Work out the finished part from the listing and answer in its coordinate system (mm). A direction names the side the tool comes from. Coordinates: 2 decimals unless noted, no trailing zeros. Write each loop counter-clockwise with the first axis right and the second up, starting at its lowest first coordinate (ties: lowest second). Pieces come first, ordered by that corner, then holes. Notation, with made-up numbers: (-15, 15) - (10, 15) arc R27 cw to (10, 52) - close; hole circle Ø6 at (45.25, 79). An arc over 180 degrees is marked (long way). Answer as a JSON object with one key per item and string values. Group by question number.
from build123d import *

# Parameters (mm, degrees)
F0_W      = 100
F0_H      = 40
F0_R      = 1.5
F1_DEPTH  = 30
F2_W      = 94
F2_H      = 34
F2_R      = 1
F3_DEPTH  = 27
F4_R      = 3
F5_DEPTH  = 5
F6_R      = 1
F7_R      = 4
F8_R      = 4
F9_R      = 6.6732690133
F10_DEPTH = 1
F11_R     = 0.99999


# Not quite as in the source:
# - a fillet or chamfer is up to 0.001 mm smaller than in the source, because OpenCascade refuses the exact size


with BuildPart() as f1:
    # F0 (on Top) → F1 (new body)
    with BuildSketch(Plane.XY):
        with Locations((-4.7806398869, -4.191e-06)):
            Rectangle(F0_W, F0_H)
        with Locations((-21.7806398869, 0)):
            Circle(F0_R, mode=Mode.SUBTRACT)
        with Locations((12.2193601131, 0)):
            Circle(F0_R, mode=Mode.SUBTRACT)
    extrude(amount=F1_DEPTH)

    # F2 (on face) → F3 (cut)
    with BuildSketch(Plane.XY.offset(30)):
        with Locations((-4.7806398869, -4.191e-06)):
            Rectangle(F2_W, F2_H)
        with Locations((-52.7806398869, 17.999995809)):
            Circle(F2_R)
        with Locations((-52.7806398869, -18.000004191)):
            Circle(F2_R)
        with Locations((43.2193601131, 17.999995809)):
            Circle(F2_R)
        with Locations((43.2193601131, -18.000004191)):
            Circle(F2_R)
    extrude(amount=-F3_DEPTH, mode=Mode.SUBTRACT)

    # F4 (on face) → F5 (cut)
    with BuildSketch(Plane.XZ.offset(20.000004191)):
        with Locations((32.2193601131, 20)):
            Circle(F4_R)
    extrude(amount=-F5_DEPTH, mode=Mode.SUBTRACT)

    # F6
    f6_edges = [f1.edges().sort_by_distance(p)[0] for p in [
        (45.21936, 19.999996, 15),
        (-4.78064, 19.999996, 0),
        (45.21936, -4e-06, 0),
        (45.21936, -20.000004, 15),
        (-4.78064, -20.000004, 0),
        (-54.78064, -4e-06, 0),
        (-54.78064, 19.999996, 15),
        (-54.78064, -20.000004, 15),
    ]]
    fillet(f6_edges, radius=F6_R)

    # F7
    f7_edges = [f1.edges().sort_by_distance(p)[0] for p in [
        (42.21936, 16.999996, 16.5),
        (-51.78064, 16.999996, 16.5),
        (-51.78064, -17.000004, 16.5),
        (42.21936, -17.000004, 16.5),
    ]]
    fillet(f7_edges, radius=F7_R)

    # F8
    f8_edges = [f1.edges().sort_by_distance(p)[0] for p in [
        (-4.78064, 16.999996, 3),
    ]]
    fillet(f8_edges, radius=F8_R)

    # F9 (on face) → F10 (cut)
    with BuildSketch(Plane.XZ.offset(20.000004191)):
        with Locations((32.2193601131, 20)):
            Circle(F9_R)
    extrude(amount=-F10_DEPTH, mode=Mode.SUBTRACT)

    # F11 (radius 1 in the source; OpenCascade refuses exactly that, so slightly less here)
    f11_edges = [f1.edges().sort_by_distance(p)[0] for p in [
        (25.546091, -19.000004, 20),
    ]]
    fillet(f11_edges, radius=F11_R)


solid = f1.part
Q1. Flat-ended cylindrical pins translate along their axes: pin 1 Ø1 at (x, y) = (-52.5, -18) entering from +Z; pin 2 Ø3.5 at (x, z) = (32.22, 20) entering from -Y. Find the tip coordinate at first contact, or state that the pin passes through.
Q2. A tool of negligible diameter and unlimited length cuts with its end or side. For faces 4 (the face through (35.08, -18.01, 20.9)), 5 (the face through (13.605, -0.575, 1.479)), 6 (the face through (-53, 18, 3)), from which of +Z, -Z, +X, -X, +Y, -Y can it reach the whole face along a straight path? Write none if from no direction.
Q3. Section A-A on y = 0 is taken. Determine the outline of the cut face in (x, z).
Q4. Consider L1, parallel to X at y = 0, z = 1.9; L2, parallel to Y at x = -18, z = 21.5; L3, parallel to X at y = -3.5, z = 18.25. Determine where each line is inside the solid, lowest interval first. Write a range as from..to.
Q5. Section B-B on z = 20 is taken. Count the separate pieces of the cut face and the enclosed holes in it, plus the area to 3 significant figures.
Q6. Section C-C on x = -41 is taken. Determine the outline of the cut face in (y, z).
Q7. Section D-D on z = 4.25 is taken. Determine the outline of the cut face in (x, y).
Q8. For a pull along Y with two mould halves and no side action, classify faces 1 (the face through (-9, -18, 30)), 2 (the face through (-5, -20, 15)), 3 (the face through (-23.28, 0.07, 1.48)) as +Y half, -Y half, draft (parallel to the pull), parting line (faces both ways), or undercut.
Numbers:
{
 "1": {"pin 1": "stops at z = 3", "pin 2": "stops at y = 17"},
 "2": {"face 4": "-Y", "face 5": "+Z, -Z", "face 6": "+Z"},
 "3": {"outline": "(-54.78, 1) arc R1 ccw to (-53.78, 0) - (-23.28, 0) - (-23.28, 3) - (-47.78, 3) arc R4 cw to (-51.78, 7) - (-51.78, 30) - (-54.78, 30) - close; (-20.28, 0) - (10.72, 0) - (10.72, 3) - (-20.28, 3) - close; (13.72, 0) - (44.22, 0) arc R1 ccw to (45.22, 1) - (45.22, 30) - (42.22, 30) - (42.22, 7) arc R4 cw to (38.22, 3) - (13.72, 3) - close"},
 "4": {"L1": "x = -54.78..-23.28, -20.28..10.72, 13.72..45.22", "L2": "y = -20..-17, 17..20", "L3": "x = -54.78..-51.78, 42.22..45.22"},
 "5": {"separate pieces": "1", "enclosed holes": "4", "area": "779 mm²"},
 "6": {"outline": "(-20, 1) arc R1 ccw to (-19, 0) - (19, 0) arc R1 ccw to (20, 1) - (20, 30) - (17, 30) - (17, 7) arc R4 cw to (13, 3) - (-13, 3) arc R4 cw to (-17, 7) - (-17, 30) - (-20, 30) - close"},
 "7": {"outline": "(-54.78, -19) arc R1 ccw to (-53.78, -20) - (44.22, -20) arc R1 ccw to (45.22, -19) - (45.22, 19) arc R1 ccw to (44.22, 20) - (-53.78, 20) arc R1 ccw to (-54.78, 19) - close; hole circle Ø2 at (-52.78, -18); hole circle Ø2 at (-52.78, 18); hole (-50.69, -13) arc R2.9 ccw to (-47.78, -15.9) - (38.22, -15.9) arc R2.9 ccw to (41.12, -13) - (41.12, 13) arc R2.9 ccw to (38.22, 15.9) - (-47.78, 15.9) arc R2.9 ccw to (-50.69, 13) - close; hole circle Ø2 at (43.22, -18); hole circle Ø2 at (43.22, 18)"},
 "8": {"face 1": "draft", "face 2": "-Y half", "face 3": "undercut"}
}
